from build123d import *

# Parameters (mm, degrees)
SKETCH_W          = 80
SKETCH_H          = 12.7
PAD_DEPTH         = 12.7
SKETCH001_R       = 2
SKETCH001_R_2     = 2.5
POCKET_DEPTH      = 6.351
POCKET_DEPTH_BACK = -6.351


with BuildPart() as part:
    # Sketch → Pad (new body)
    with BuildSketch(Plane.XY):
        Rectangle(SKETCH_W, SKETCH_H)
        with BuildLine():
            ThreePointArc((0, -4.898979), (8, 0), (0, 4.898979))
            ThreePointArc((0, 4.898979), (-8, 0), (0, -4.898979))
        make_face(mode=Mode.SUBTRACT)
    extrude(amount=PAD_DEPTH)

    # Sketch001 → Pocket (cut, two sides)
    with BuildSketch(Plane.XZ) as pocket_sk:
        with Locations((-35, 6.35)):
            Circle(SKETCH001_R)
        with Locations((-20, 6.35)):
            Circle(SKETCH001_R)
        with Locations((20, 6.35)):
            Circle(SKETCH001_R_2)
        with Locations((35, 6.35)):
            Circle(SKETCH001_R_2)
    extrude(amount=-POCKET_DEPTH, mode=Mode.SUBTRACT)
    extrude(pocket_sk.sketch, amount=-POCKET_DEPTH_BACK, mode=Mode.SUBTRACT)


solid = part.part
CAD build for the part. Positions are in the model's coordinates, mm. Give positions to 0.01 mm unless a question says otherwise; leave off trailing zeros. Loops run counter-clockwise (first coordinate to the right, second up) from the corner with the lowest first, then second, coordinate; pieces in that order, holes last. Notation, with made-up numbers: M -34.75,26 L -17.75,26 A11 ccw -17.75,46 Z; hole C 29.5,7 d2. An arc over 180 degrees is marked long. Answer in a Markdown table with one row per item. Add a question column.
Item 1: Band-saw the part on B-B on y = 1. Give the cut face in (x, z).
Item 2: Band-saw the part on D-D on z = 2. Give the cut face in (x, y), then the cut area to 3 significant figures.
Item 3: Mould opens along Y. For faces 1 (the face through (8, 0, 6)), 2 (the face through (-8, 0, 6)), 3 (the face through (40, 0, 6)), 4 (the face through (-1, 6.35, 6)) say: +Y half, -Y half, draft (parallel to the pull), parting line (faces both ways), or undercut.
Item 4: Probe probe 1 along Z at (x, y) = (-35, -2.5); probe 2 along Z at (x, y) = (20, -3.5); probe 3 along X at (y, z) = (-0.75, 6.75). List the from-to ranges inside material, lowest first.
Item 5: Band-saw the part on A-A on x = -20. Give the cut face in (y, z).
Item 6: Band-saw the part on C-C on z = 6.35. Give the cut face in (x, y).
Item 7: Drop a flat-ended pin along its axis: P1, Ø2.5, axis at x = -35, z = 6.35, coming from the -Y side. Give the stop position or say it passes through.
Reply:
| question | item | result |
|---|---|---|
| 1 | outline | M -40,0 L -7.91,0 L -7.91,12.7 L -40,12.7 Z; M 7.91,0 L 40,0 L 40,12.7 L 7.91,12.7 Z; hole C -35,6.35 d4; hole C -20,6.35 d4; hole C 20,6.35 d5; hole C 35,6.35 d5 |
| 2 | outline | M -40,-6.35 L 40,-6.35 L 40,6.35 L -40,6.35 Z; hole M 0,-4.9 A5.5 ccw long 0,4.9 A5.5 ccw long Z |
| 2 | area | 868 mm^2 |
| 3 | face 1 | undercut |
| 3 | face 2 | undercut |
| 3 | face 3 | draft |
| 3 | face 4 | +Y half |
| 4 | probe 1 | z = 0 to 4.35, 8.35 to 12.7 |
| 4 | probe 2 | z = 0 to 3.85, 8.85 to 12.7 |
| 4 | probe 3 | x = -40 to -36.96, -33.04 to -21.96, -18.04 to -7.95, 7.95 to 17.53, 22.47 to 32.53, 37.47 to 40 |
| 5 | outline | M -6.35,0 L 6.35,0 L 6.35,4.35 L -6.35,4.35 Z; M -6.35,8.35 L 6.35,8.35 L 6.35,12.7 L -6.35,12.7 Z |
| 6 | outline | M -40,-6.35 L -37,-6.35 L -37,6.35 L -40,6.35 Z; M -33,-6.35 L -22,-6.35 L -22,6.35 L -33,6.35 Z; M -18,-6.35 L 17.5,-6.35 L 17.5,6.35 L -18,6.35 Z; M 22.5,-6.35 L 32.5,-6.35 L 32.5,6.35 L 22.5,6.35 Z; M 37.5,-6.35 L 40,-6.35 L 40,6.35 L 37.5,6.35 Z; hole M 0,-4.9 A5.5 ccw long 0,4.9 A5.5 ccw long Z |
| 7 | P1 | passes through |
